CAD build for the part. Positions are in the model's coordinates, mm. A direction names the side the tool comes from. Coordinates: 2 decimals unless noted, no trailing zeros. Order: outer loops, then holes, each group sorted by start corner. A loop starts at its lowest first (then second) coordinate and runs counter-clockwise, first axis right, second up. Notation, with made-up numbers: M 86.5,6.5 L 125.5,6.5 A21 ccw 125.5,13.5 Z; hole C 0.25,42 d2. An arc over 180 degrees is marked long. Write item = value, one per line.
from build123d import *

# Parameters (mm, degrees)
F1_DEPTH = 90
F2_DEPTH = 75
F3_R     = 10
F4_DEPTH = 125
F6_D     = 17.5
F6_DEPTH = 200
F6_TIP   = 5.2575304165


with BuildPart() as f1:
    # F0 (on Front) → F1 (new body, symmetric)
    with BuildSketch(Plane.XZ):
        with BuildLine():
            ThreePointArc((-38.5871816571, 95.6880305716), (0, 85), (38.5871816571, 95.6880305716))
            ThreePointArc((38.5871816571, 95.6880305716), (65.2649930065, 123.0475888762), (75, 160))
            ThreePointArc((75, 160), (-36.9524111238, 225.2649930065), (-38.5871816571, 95.6880305716))
        make_face()
    extrude(amount=F1_DEPTH, both=True)

    # F0 (on Front) → F2 (join, symmetric)
    with BuildSketch(Plane.XZ):
        Polygon((-90, -10), (90, -10), (90, 10), (50, 10), (0, 10), (-50, 10), (-90, 10), align=None)
        with BuildLine():
            Line((50, 10), (90, 10))
            add(Edge.make_bspline(
                [(90, 10), (74.3035884973, 18.2071101409), (58.6071769946, 26.4142202817), (50, 40)],
                knots=[0, 0, 0, 0, 0.4839662752, 0.4839662752, 0.4839662752, 0.4839662752], degree=3))
            Line((50, 40), (50, 10))
        make_face()
        with BuildLine():
            add(Edge.make_bspline(
                [(-90, 10), (-74.3035884973, 18.2071101409), (-58.6071769946, 26.4142202817), (-50, 40)],
                knots=[0, 0, 0, 0, 0.4839662752, 0.4839662752, 0.4839662752, 0.4839662752], degree=3))
            Line((-90, 10), (-50, 10))
            Line((-50, 10), (-50, 40))
        make_face()
        with BuildLine():
            Line((0, 10), (50, 10))
            Line((50, 10), (50, 40))
            add(Edge.make_bspline(
                [(50, 40), (40.8225142283, 54.4859691093), (39.7048479427, 75.0869998404), (38.5871816571, 95.6880305716)],
                knots=[0.4839662752, 0.4839662752, 0.4839662752, 0.4839662752, 1, 1, 1, 1], degree=3))
            ThreePointArc((38.5871816571, 95.6880305716), (0, 85), (-38.5871816571, 95.6880305716))
            add(Edge.make_bspline(
                [(-50, 40), (-40.8225142283, 54.4859691093), (-39.7048479427, 75.0869998404), (-38.5871816571, 95.6880305716)],
                knots=[0.4839662752, 0.4839662752, 0.4839662752, 0.4839662752, 1, 1, 1, 1], degree=3))
            Line((-50, 40), (-50, 10))
            Line((-50, 10), (0, 10))
        make_face()
        with BuildLine():
            ThreePointArc((-38.5871816571, 95.6880305716), (0, 85), (38.5871816571, 95.6880305716))
            ThreePointArc((38.5871816571, 95.6880305716), (65.2649930065, 123.0475888762), (75, 160))
            ThreePointArc((75, 160), (-36.9524111238, 225.2649930065), (-38.5871816571, 95.6880305716))
        make_face()
    extrude(amount=F2_DEPTH, both=True)

    # F3 (on face) → F4 (join)
    with BuildSketch(Plane.XZ.offset(90)):
        with Locations((0, 160)):
            Circle(F3_R)
    extrude(amount=F4_DEPTH)

    # F6
    with Locations(Plane(origin=(0, 0, -10), x_dir=(1, 0, 0), z_dir=(0, 0, -1))):
        with Locations((0, 0)):
            Hole(F6_D / 2, depth=F6_DEPTH)
            with Locations((0, 0, -(F6_DEPTH + F6_TIP / 2))):  # 118° drill point
                Cone(0, F6_D / 2, F6_TIP, mode=Mode.SUBTRACT)


solid = f1.part
(1) Slice it at D-D, the plane y = -154.5. Write the cut outline in (x, z), then the cut area to 3 significant figures.
Evaluation:
outline = C 0,160 d20
area = 314 mm²
(2) Slice it at B-B, the plane x = -17.5. Write the cut outline in (y, z).
Evaluation:
outline = M -90,87.07 L -75,87.07 L -75,-10 L 75,-10 L 75,87.07 L 90,87.07 L 90,232.93 L -90,232.93 Z
(3) Tool access for faces 5 (the face through (-1, 90, 161)), 6 (the face through (-2.17, -151.62, 150.24)): list every direction of +Z, -Z, +X, -X, +Y, -Y with a clear straight run to the whole face (end or side of a thin tool).
Evaluation:
face_5 = +Z, -Z, +X, -X, +Y
face_6 = -Y
(4) Wall check: line 1 (Y direction, x = 0, z = 68); line 2 (Y direction, x = -0.5, z = 187); line 3 (Y direction, x = -25, z = 83). Give the ranges that are in metal, low to high. Write a range as from..to.
Evaluation:
line_1 = -75..-8.75, 8.75..75
line_2 = -90..-8.74, 8.74..90
line_3 = -75..75
(5) Slice it at A-A, the plane z = 160. Write the cut outline in (x, y).
Evaluation:
outline = M -75,-90 L -10,-90 L -10,-215 L 10,-215 L 10,-90 L 75,-90 L 75,90 L -75,90 Z; hole C 0,0 d17.5
(6) Pin check, flat tips, straight feed: pin 1 Ø6 at (y, z) = (-26, 118) entering from -X; pin 2 Ø5 at (x, y) = (-59, -78) entering from -Z; pin 3 Ø1 at (y, z) = (31.5, 96.5) entering from +X. Stop position of each tip, or through.
Evaluation:
pin_1 = -64.06
pin_2 = 110.68
pin_3 = 40.69
(7) Slice it at C-C, the plane z = 115. Write the cut outline in (x, y).
Evaluation:
outline = M -60,-90 L 60,-90 L 60,90 L -60,90 Z; hole C 0,0 d17.5
(8) Pull direction X, two halves, no side cores. Call faces 1 (the face through (0, -215, 160)), 2 (the face through (-90, -1, 0)), 3 (the face through (6.944, 5.324, 91.4)), 4 (the face through (-0.329, 1.483, 194.344)): +X half, -X half, draft (parallel to the pull), parting line (faces both ways), or undercut.
Evaluation:
face_1 = draft
face_2 = -X half
face_3 = undercut
face_4 = undercut
